from build123d import *

# Parameters (mm, degrees)
CHANFREIN1_SIZE = 0.25
CHANFREIN3_SIZE = 0.5
CONG_1_R        = 0.5


with BuildPart() as part:
    # Esquisse1 → Base-Révolution (revolve)
    with BuildSketch(Plane.XY, mode=Mode.PRIVATE) as base_r_volution_sk:
        Polygon((0, 0), (0, 3), (-25, 3), (-25, 10), (-55, 10), (-55, 0), align=None)
    revolve(base_r_volution_sk.sketch.rotate(Axis((-58.669915368, 0, 0), (1, 0, 0)), 90), axis=Axis((-58.669915368, 0, 0), (1, 0, 0)))

    # Chanfrein1
    chanfrein1_edges = [part.edges().sort_by_distance(p)[0] for p in [
        (0, 0, -3),
    ]]
    chamfer(chanfrein1_edges, length=CHANFREIN1_SIZE)

    # Chanfrein3
    chanfrein3_edges = [part.edges().sort_by_distance(p)[0] for p in [
        (-55, 0, -10),
        (-25, 0, -10),
    ]]
    chamfer(chanfrein3_edges, length=CHANFREIN3_SIZE)

    # Congé1
    cong_1_edges = [part.edges().sort_by_distance(p)[0] for p in [
        (-25, 0, -3),
    ]]
    fillet(cong_1_edges, radius=CONG_1_R)


solid = part.part
Source: CAD feature listing. Evaluate the final solid. Frame: model axes, mm. A direction names the side the tool comes from. Round coordinates to 2 decimals unless told otherwise and drop trailing zeros. Loops run counter-clockwise (first coordinate to the right, second up) from the corner with the lowest first, then second, coordinate; pieces in that order, holes last. Notation, with made-up numbers: M 64.5,9 L 122.5,9 A15 cw 122.5,28 Z; hole C 74.25,-28.5 d11. An arc over 180 degrees is marked long. Return JSON: item names as keys, results as strings. Group by question number.
1. Section query C-C on x = -22. Output: boundary loops of the cut face in (y, z).
2. Reachability of faces 1 (the face through (-55, 0, 0)), 2 (the face through (-12.54, -0.9, 2.86)) from +Z, -Z, +X, -X, +Y, -Y: full face, straight path, thin tool, end or side. Return the list, or none.
3. Section query D-D on x = -47. Output: boundary loops of the cut face in (y, z), and give its area (3 significant figures).
4. Pin query (flat end, axial travel): pin 1 (5 mm diameter, centred on x = -49, z = -6, fed in from -Y); pin 2 (8 mm diameter, centred on x = -25, y = -7, fed in from +Z); pin 3 (10 mm diameter, centred on x = -30.5, y = 5.5, fed in from -Z). Return the tip coordinate at first contact, or that it passes through.
5. Section query A-A on y = 0. Output: boundary loops of the cut face in (x, z), and give its area (3 significant figures).
6. Material intervals for line 1 along X through (y, z) = (4.25, -1.5); line 2 along X through (y, z) = (6.75, 7); line 3 along Z through (x, y) = (-35, -1.75), sorted ascending. Write a range as from..to.
Checks:
{
 "1": {"outline": "C 0,0 d6"},
 "2": {"face 1": "+Z, -Z, -X, +Y, -Y", "face 2": "+X"},
 "3": {"outline": "C 0,0 d20", "area": "314 mm²"},
 "4": {"pin 1": "stops at y = -9.37", "pin 2": "stops at z = 9.53", "pin 3": "stops at z = -9.99"},
 "5": {"outline": "M -55,-9.5 L -54.5,-10 L -25.5,-10 L -25,-9.5 L -25,-3.5 A0.5 cw -24.5,-3 L -0.25,-3 L 0,-2.75 L 0,2.75 L -0.25,3 L -24.5,3 A0.5 cw -25,3.5 L -25,9.5 L -25.5,10 L -54.5,10 L -55,9.5 Z", "area": "750 mm²"},
 "6": {"line 1": "x = -55..-25", "line 2": "x = -54.78..-25.22", "line 3": "z = -9.85..9.85"}
}
